```python
from build123d import *

# Parameters (mm, degrees)
BOSS_EXTRUDE1_DEPTH   = 4.7625
F_6_CLEARANCE_HOLE1_D = 4.3053
SKETCH5_R             = 9.525
CUT_EXTRUDE1_DEPTH    = 5.7625


with BuildPart() as part:
    # Sketch1 → Boss-Extrude1 (new body)
    with BuildSketch(Plane.XY.offset(-34.431186078)):
        with BuildLine():
            Line((-842.127056947, 5946.106287623), (-962.650056947, 5946.106287623))
            ThreePointArc((-962.650056947, 5946.106287623), (-963.727687681, 5945.659918357), (-964.174056947, 5944.582287623))
            Line((-964.174056947, 5944.582287623), (-964.174056947, 5932.612537623))
            ThreePointArc((-964.174056947, 5932.612537623), (-966.033928886, 5928.122409562), (-970.524056947, 5926.262537623))
            Line((-970.524056947, 5926.262537623), (-973.095806947, 5926.262537623))
            ThreePointArc((-973.095806947, 5926.262537623), (-974.173437681, 5925.816168357), (-974.619806947, 5924.738537623))
            Line((-974.619806947, 5924.738537623), (-974.619806947, 5915.392415905))
            ThreePointArc((-974.619806947, 5915.392415905), (-974.372123334, 5914.559593907), (-973.709580595, 5913.997475796))
            Line((-973.709580595, 5913.997475796), (-899.073125038, 5881.157435351))
            ThreePointArc((-899.073125038, 5881.157435351), (-898.178349327, 5881.054505693), (-897.381720655, 5881.474744726))
            Line((-897.381720655, 5881.474744726), (-876.633992352, 5902.222473029))
            ThreePointArc((-876.633992352, 5902.222473029), (-853.601284124, 5907.100841083), (-839.803970731, 5888.023674985))
            ThreePointArc((-839.803970731, 5888.023674985), (-839.332483448, 5886.99508367), (-838.281835234, 5886.575037623))
            Line((-838.281835234, 5886.575037623), (-831.681306947, 5886.575037623))
            ThreePointArc((-831.681306947, 5886.575037623), (-830.603676212, 5887.021406888), (-830.157306947, 5888.099037623))
            Line((-830.157306947, 5888.099037623), (-830.157306947, 5924.738537623))
            ThreePointArc((-830.157306947, 5924.738537623), (-830.603676212, 5925.816168357), (-831.681306947, 5926.262537623))
            Line((-831.681306947, 5926.262537623), (-834.253056947, 5926.262537623))
            ThreePointArc((-834.253056947, 5926.262537623), (-838.743185007, 5928.122409562), (-840.603056947, 5932.612537623))
            Line((-840.603056947, 5932.612537623), (-840.603056947, 5944.582287623))
            ThreePointArc((-840.603056947, 5944.582287623), (-841.049426212, 5945.659918357), (-842.127056947, 5946.106287623))
        make_face()
    extrude(amount=BOSS_EXTRUDE1_DEPTH)

    # #6 Clearance Hole1 (through all)
    with Locations(Plane.XY.offset(-29.668686078)):
        with Locations((-840.539556947, 5918.325037623), (-889.688556947, 5900.862537623), (-928.423556947, 5932.612537623)):
            Hole(F_6_CLEARANCE_HOLE1_D / 2)

    # Sketch5 → Cut-Extrude1 (cut, through all)
    with BuildSketch(Plane.XY.offset(-29.668686078)):
        with Locations((-857.938556947, 5927.524153596)):
            Circle(SKETCH5_R)
        with Locations((-902.388556947, 5927.342037623)):
            Circle(SKETCH5_R)
        with Locations((-946.838556947, 5927.342037623)):
            Circle(SKETCH5_R)
    extrude(amount=-CUT_EXTRUDE1_DEPTH, mode=Mode.SUBTRACT)


solid = part.part
```
Here's how the part is built. I have some questions about the finished solid (model axes, mm). A direction names the side the tool comes from. Coordinates: 2 decimals unless noted, no trailing zeros. Loops run counter-clockwise (first coordinate to the right, second up) from the corner with the lowest first, then second, coordinate; pieces in that order, holes last. Notation, with made-up numbers: (-35, 45.25) -> (22, 45.25) arc R21 ccw to (22, 60.25) -> close; hole circle Ø1 at (32.25, 39.25). An arc over 180 degrees is marked (long way). Return JSON: item names as keys, results as strings.
1) If we section it at D-D, the plane y = 5912.5: Write out the boundary of the cut face in (x, z).
Results below:
{"outline": "(-970.31, -34.43) -> (-830.16, -34.43) -> (-830.16, -29.67) -> (-970.31, -29.67) -> close"}
2) For faces 5 (the face through (-887.153, 5891.703, -32.083)), 6 (the face through (-840.073, 5916.224, -32.083)), 7 (the face through (-840.603, 5939, -32)), which set-ups out of +Z, -Z, +X, -X, +Y, -Y let a thin tool reach every point of the face, with its end or its side?
Results below:
{"face 5": "+Z, -Z, -Y", "face 6": "+Z, -Z", "face 7": "+Z, -Z, +X, +Y"}
3) I need wall thicknesses on line 1 (X direction, y = 5928, z = -34.15); line 2 (X direction, y = 5927, z = -31.55); line 3 (Y direction, x = -853, z = -30.05). Which ranges of each line are inside material? Lowest first, please. Write a range as from..to.
Results below:
{"line 1": "-966.16..-956.34, -937.34..-911.89, -892.89..-867.45, -848.43..-838.62", "line 2": "-967.55..-956.36, -937.32..-911.91, -892.87..-867.45, -848.43..-837.22", "line 3": "5906.86..5919.38, 5935.67..5946.11"}
4) If we section it at A-A, the plane x = -903.5: Write out the boundary of the cut face in (y, z), then the cut area to 3 significant figures.
Results below:
{"outline": "(5883.11, -34.43) -> (5917.88, -34.43) -> (5917.88, -29.67) -> (5883.11, -29.67) -> close; (5936.8, -34.43) -> (5946.11, -34.43) -> (5946.11, -29.67) -> (5936.8, -29.67) -> close", "area": "210 mm²"}
5) If we section it at B-B, the plane z = -31.75: Write out the boundary of the cut face in (x, y) (3 decimals).
Results below:
{"outline": "(-974.62, 5915.392) arc R1.524 ccw to (-973.71, 5913.997) -> (-899.073, 5881.157) arc R1.524 ccw to (-897.382, 5881.475) -> (-876.634, 5902.222) arc R21.59 cw to (-839.804, 5888.024) arc R1.524 ccw to (-838.282, 5886.575) -> (-831.681, 5886.575) arc R1.524 ccw to (-830.157, 5888.099) -> (-830.157, 5924.739) arc R1.524 ccw to (-831.681, 5926.263) -> (-834.253, 5926.263) arc R6.35 cw to (-840.603, 5932.613) -> (-840.603, 5944.582) arc R1.524 ccw to (-842.127, 5946.106) -> (-962.65, 5946.106) arc R1.524 ccw to (-964.174, 5944.582) -> (-964.174, 5932.613) arc R6.35 cw to (-970.524, 5926.263) -> (-973.096, 5926.263) arc R1.524 ccw to (-974.62, 5924.739) -> close; hole circle Ø19.05 at (-946.839, 5927.342); hole circle Ø4.305 at (-928.424, 5932.613); hole circle Ø19.05 at (-902.389, 5927.342); hole circle Ø4.305 at (-889.689, 5900.863); hole circle Ø19.05 at (-857.939, 5927.524); hole circle Ø4.305 at (-840.54, 5918.325)"}
6) If we section it at C-C, the plane x = -852: Write out the boundary of the cut face in (y, z).
Results below:
{"outline": "(5906.41, -34.43) -> (5920.08, -34.43) -> (5920.08, -29.67) -> (5906.41, -29.67) -> close; (5934.97, -34.43) -> (5946.11, -34.43) -> (5946.11, -29.67) -> (5934.97, -29.67) -> close"}
7) Will these pins go through, and if not, where does the flat tip stop? pin 1 (17 mm diameter, centred on x = -857.94, y = 5927.52, fed in from +Z); pin 2 (0.8 mm diameter, centred on x = -972, z = -33, fed in from +Y); pin 3 (1.4 mm diameter, centred on x = -833.5, z = -31.5, fed in from -Y); pin 4 (2.5 mm diameter, centred on y = 5936, z = -32, fed in from -X).
Results below:
{"pin 1": "through", "pin 2": "y = 5926.26", "pin 3": "y = 5886.58", "pin 4": "x = -964.17"}
8) Thinking about a two-plate mould opening in X: for faces 1 (the face through (-929.417, 5930.703, -32.083)), 2 (the face through (-964.174, 5939, -32)), 3 (the face through (-830.157, 5906, -32)), 4 (the face through (-853.928, 5907.224, -32.083)), which applies, +X half, -X half, draft (parallel to the pull), parting line (faces both ways), or undercut?
Results below:
{"face 1": "undercut", "face 2": "-X half", "face 3": "+X half", "face 4": "undercut"}
